Part model, mm, in its own coordinate system. Give positions to 0.01 mm unless a question says otherwise; leave off trailing zeros. Write item = value, one per line. Start each with the question number.
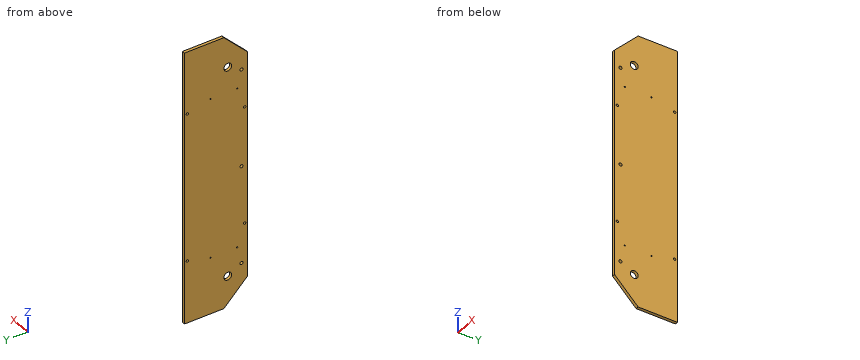
Autodesk Inventor part; units mm, degrees
ref_plane "YZ Plane" through (0, 0, 0) normal (1, 0, 0) x (0, 1, 0)
ref_plane "XZ Plane" through (0, 0, 0) normal (0, 1, 0) x (-1, 0, 0)
ref_plane "XY Plane" through (0, 0, 0) normal (0, 0, 1) x (1, 0, 0)
sketch "Sketch1" plane through (0, 0, 0) normal (1, 0, 0) x (0, 1, 0)
  line L0 (0, 0) -> (101.6, 0)
  line L1 (101.6, 0) -> (101.6, -444.5)
  line L2 (101.6, -444.5) -> (0, -444.5)
  line L3 (0, -444.5) -> (0, 0)
  circle A0 centre (31.75, -50.8) radius 6.3627
  circle A1 centre (31.75, -393.7) radius 6.3627
  circle A2 centre (86.2838, -165.5318) radius 1.5875
  circle A3 centre (70.2818, -165.5318) radius 1.5875
  circle A4 centre (15.3162, -278.9682) radius 1.5875
  circle A5 centre (31.3182, -278.9682) radius 1.5875
  dimension "d0" = 101.6
  dimension "d1" = 444.5
  dimension "d2" = 12.7254
  dimension "d3" = 31.75
  dimension "d4" = 50.8
  dimension "d5" = 50.8
  dimension "d22" = 165.5318
  dimension "d23" = 3.175
  dimension "d24" = 15.3162
  dimension "d25" = 3.175
  dimension "d26" = 16.002
  dimension "d27" = 165.5318
  dimension "d28" = 3.175
  dimension "d29" = 15.3162
  dimension "d30" = 165.5318
  dimension "d31" = 3.175
  dimension "d32" = 16.002
  dimension "d33" = 165.5318
extrude "Extrusion1" add sketch "Sketch1" along normal blind 4.7625 contours L0 L1 L2 L3 | A2 | A3 | A4 | A5
chamfer "Chamfer1" distance 38.1 angle 45 1 edges at (2.3813, 0, 0)
chamfer "Chamfer2" distance 38.1 angle 45 1 edges at (2.3813, 0, -444.5)
sketch "Sketch7" plane through (4.7625, 0, 0) normal (1, 0, 0) x (0, 0, -1)
  line L0 (444.5, 38.1) -> (406.4, 0)
  line L1 (444.5, 38.1) -> (444.5, 101.6)
  line L2 (444.5, 101.6) -> (0, 101.6)
  line L3 (0, 101.6) -> (0, 38.1)
  line L4 (38.1, 0) -> (0, 38.1)
  line L5 (38.1, 0) -> (406.4, 0)
  circle A0 centre (393.7, 31.75) radius 6.3627
  circle A1 centre (50.8, 31.75) radius 6.3627
  point P0 (0, 0)
  point P1 (101.6, 97.155)
  point P2 (342.9, 97.155)
  point P3 (127, 4.445)
  point P4 (317.5, 4.445)
  dimension "d95" = 4.445
  dimension "d96" = 4.445
  dimension "d97" = 4.445
  dimension "d98" = 4.445
  dimension "d99" = 101.6
  dimension "d100" = 101.6
  dimension "d101" = 127
  dimension "d102" = 127
hole "Hole2" at (4.7625, 97.155, -101.6) at (4.7625, 97.155, -342.9) at (4.7625, 4.445, -127) at (4.7625, 4.445, -317.5) direction (-1, 0, 0) diameter 3.81 depth 25.4 tip angle 118
sketch "Sketch9" plane through (4.7625, 0, 0) normal (1, 0, 0) x (0, 0, -1)
  line L0 (444.5, 38.1) -> (444.5, 101.6)
  line L1 (38.1, 0) -> (406.4, 0)
  line L2 (0, 101.6) -> (0, 38.1)
  point P0 (0, 0)
  point P1 (352.425, 59.69)
  point P2 (352.425, 16.51)
  point P3 (92.075, 16.51)
  point P4 (92.075, 59.69)
  dimension "d115" = 43.18
  dimension "d116" = 92.075
  dimension "d117" = 92.075
  dimension "d118" = 16.51
  dimension "d119" = 92.075
  dimension "d120" = 92.075
  dimension "d121" = 43.18
  dimension "d122" = 16.51
hole "Hole3" at (4.7625, 59.69, -352.425) at (4.7625, 16.51, -352.425) at (4.7625, 16.51, -92.075) at (4.7625, 59.69, -92.075) direction (-1, 0, 0) diameter 2.032 depth 7.6708 tip angle 118
sketch "Sketch10" plane through (4.7625, 0, 0) normal (1, 0, 0) x (0, 0, -1)
  line L0 (38.1, 0) -> (406.4, 0)
  line L1 (0, 101.6) -> (0, 38.1)
  line L2 (444.5, 38.1) -> (444.5, 101.6)
  point P0 (0, 0)
  point P1 (63.5, 9.525)
  point P2 (222.25, 9.525)
  point P3 (381, 9.525)
  dimension "d130" = 9.525
  dimension "d131" = 63.5
  dimension "d132" = 63.5
  dimension "d133" = 317.5
  dimension "d134" = 158.75
  dimension "d135" = 9.525
hole "Hole4" at (4.7625, 9.525, -63.5) at (4.7625, 9.525, -222.25) at (4.7625, 9.525, -381) direction (-1, 0, 0) diameter 5.08 depth 19.05 tip angle 118
properties part number "DriveTrain3.0" material "Aluminum 6061"
Q1. Slice it at A-A (x = 3.5). Give the number of separate pieces and of enclosed holes in the cut face, and give its area (3 significant figures).
Q2. Probe line 1 along Z through (x, y) = (1.9, 59.69); line 2 along Z through (x, y) = (1.85, 31.5); line 3 along Y through (x, z) = (2.55, -127). List the from-to ranges inside material, lowest first.
Q3. Drop flat-ended pins along their axis: P1, Ø7.5, axis at y = 31.75, z = -50.8, coming from the -X side; P2, Ø1.5, axis at x = 4, y = 36, coming from the -Z side. Give the stop position or say it passes through.
Working result:
q1.separate_pieces = 1
q1.enclosed_holes = 13
q1.area = 43,300 mm2
q2.line_1 = -444.5 to -353.44, -351.41 to -93.09, -91.06 to 0
q2.line_2 = -437.9 to -400.06, -387.34 to -57.16, -44.44 to -6.6
q2.line_3 = 0 to 2.54, 6.35 to 101.6
q3.P1 = through
q3.P2 = -443.15
